from build123d import *

# Parameters (mm, degrees)
ESBO_O1_R                = 2.75
ESBO_O1_R_2              = 1.75
RESSALTO_EXTRUS_O1_DEPTH = 1
ESBO_O1_3_R              = 2.75
ESBO_O1_3_R_2            = 1.75
RESSALTO_EXTRUS_O2_DEPTH = 5
ESBO_O2_W                = 7
ESBO_O2_H                = 25
CORTE_EXTRUS_O1_DEPTH    = 6
CORTE_EXTRUS_O2_DEPTH    = 6
ESBO_O4_W                = 4
ESBO_O4_H                = 4
RESSALTO_EXTRUS_O3_DEPTH = 2


with BuildPart() as part:
    # Esboço1 → Ressalto-extrusão1 (new body)
    with BuildSketch(Plane.XY):
        with BuildLine():
            Line((23.75, 18.5), (-23.75, 18.5))
            ThreePointArc((-23.75, 18.5), (-21.805456352, 17.694543648), (-21, 15.75))
            ThreePointArc((-21, 15.75), (-23.75, 13), (-26.5, 15.75))
            Line((-26.5, 15.75), (-26.5, -15.75))
            ThreePointArc((-26.5, -15.75), (-23.75, -13), (-21, -15.75))
            ThreePointArc((-21, -15.75), (-21.805456352, -17.694543648), (-23.75, -18.5))
            Line((-23.75, -18.5), (23.75, -18.5))
            ThreePointArc((23.75, -18.5), (21.805456352, -13.805456352), (26.5, -15.75))
            Line((26.5, -15.75), (26.5, 15.75))
            ThreePointArc((26.5, 15.75), (21.805456352, 13.805456352), (23.75, 18.5))
        make_face()
        with Locations((23.75, 15.75)):
            Circle(ESBO_O1_R)
        with Locations((23.75, 15.75)):
            Circle(ESBO_O1_R_2, mode=Mode.SUBTRACT)
        with Locations((23.75, -15.75)):
            Circle(ESBO_O1_R)
        with Locations((23.75, -15.75)):
            Circle(ESBO_O1_R_2, mode=Mode.SUBTRACT)
        with Locations((-23.75, -15.75)):
            Circle(ESBO_O1_R)
        with Locations((-23.75, -15.75)):
            Circle(ESBO_O1_R_2, mode=Mode.SUBTRACT)
        with Locations((-23.75, 15.75)):
            Circle(ESBO_O1_R)
        with Locations((-23.75, 15.75)):
            Circle(ESBO_O1_R_2, mode=Mode.SUBTRACT)
    extrude(amount=RESSALTO_EXTRUS_O1_DEPTH)

    # Esboço1<3> → Ressalto-extrusão2 (add)
    with BuildSketch(Plane.XY):
        with Locations((-23.75, 15.75)):
            Circle(ESBO_O1_3_R)
        with Locations((-23.75, 15.75)):
            Circle(ESBO_O1_3_R_2, mode=Mode.SUBTRACT)
        with Locations((23.75, 15.75)):
            Circle(ESBO_O1_3_R)
        with Locations((23.75, 15.75)):
            Circle(ESBO_O1_3_R_2, mode=Mode.SUBTRACT)
        with Locations((23.75, -15.75)):
            Circle(ESBO_O1_3_R)
        with Locations((23.75, -15.75)):
            Circle(ESBO_O1_3_R_2, mode=Mode.SUBTRACT)
        with Locations((-23.75, -15.75)):
            Circle(ESBO_O1_3_R)
        with Locations((-23.75, -15.75)):
            Circle(ESBO_O1_3_R_2, mode=Mode.SUBTRACT)
    extrude(amount=RESSALTO_EXTRUS_O2_DEPTH)

    # Esboço2 → Corte-extrusão1 (cut)
    with BuildSketch(Plane.XY.offset(1)):
        with Locations((23, 0)):
            Rectangle(ESBO_O2_W, ESBO_O2_H)
    extrude(amount=-CORTE_EXTRUS_O1_DEPTH, mode=Mode.SUBTRACT)

    # Esboço3 → Corte-extrusão2 (cut)
    with BuildSketch(Plane(origin=(0, 0, 0), x_dir=(-1, 0, 0), z_dir=(0, 0, -1))):
        with BuildLine():
            Line((7.25, 12.814331343), (18.75, 12.814331343))
            Line((18.75, 12.814331343), (18.75, 8.814331343))
            Line((18.75, 8.814331343), (7.25, 8.814331343))
            ThreePointArc((7.25, 8.814331343), (6.75, 8.314331343), (7.25, 7.814331343))
            Line((7.25, 7.814331343), (19.75, 7.814331343))
            Line((19.75, 7.814331343), (19.75, 13.814331343))
            Line((19.75, 13.814331343), (7.25, 13.814331343))
            ThreePointArc((7.25, 13.814331343), (6.75, 13.314331343), (7.25, 12.814331343))
        make_face()
    extrude(amount=-CORTE_EXTRUS_O2_DEPTH, mode=Mode.SUBTRACT)

    # Esboço4 → Ressalto-extrusão3 (add)
    with BuildSketch(Plane.XY.offset(1)):
        with Locations((-16.75, 10.814331343)):
            Rectangle(ESBO_O4_W, ESBO_O4_H)
    extrude(amount=RESSALTO_EXTRUS_O3_DEPTH)


solid = part.part
Read the model definition and answer for the solid it produces. Units are mm, in the model's axes. A direction names the side the tool comes from. Coordinates: 2 decimals unless noted, no trailing zeros. Order: outer loops, then holes, each group sorted by start corner. A loop starts at its lowest first (then second) coordinate and runs counter-clockwise, first axis right, second up. Notation, with made-up numbers: (17.5, 29.5) -> (75.5, 29.5) arc R19 ccw to (75.5, 55.5) -> close; hole circle Ø10 at (-5, -26). An arc over 180 degrees is marked (long way). Answer as a JSON object with one key per item and string values.
1) A tool of negligible diameter and unlimited length cuts with its end or side. For faces 1 (the face through (23, -12.5, 0.5)), 2 (the face through (26.5, 14.1, 0.5)), 3 (the face through (-18.75, 11, 1)), 4 (the face through (-22, 15, 5)), 5 (the face through (-14.75, 11, 2)), from which of +Z, -Z, +X, -X, +Y, -Y can it reach the whole face along a straight path? Write none if from no direction.
Model answer:
{"face 1": "+Z, -Z, +X", "face 2": "+Z, -Z, +X, +Y, -Y", "face 3": "+Z, -Z", "face 4": "+Z, +X, -X, +Y, -Y", "face 5": "+Z, +X, +Y, -Y"}
2) Each of these flat-tipped pins is pushed along its axis until it touches: pin 1 (3 mm diameter, centred on x = -17.5, y = 11.5, fed in from +Z); pin 2 (1.1 mm diameter, centred on y = 10.5, z = 0.5, fed in from +X); pin 3 (1.5 mm diameter, centred on x = -10.5, z = 2, fed in from -Y); pin 4 (3 mm diameter, centred on x = 12, y = 7.5, fed in from +Z). Where does it stop, or does it pass through?
Model answer:
{"pin 1": "stops at z = 3", "pin 2": "stops at x = 19.5", "pin 3": "passes through", "pin 4": "stops at z = 1"}
3) A cutting plane is placed at A-A, the plane z = 2. State how many separate pieces and enclosed holes the cut face has, plus the area to 3 significant figures.
Model answer:
{"separate pieces": "5", "enclosed holes": "4", "area": "72.5 mm²"}
4) Consider line 1 along Y through (x, z) = (-23.75, 1.1); line 2 along Y through (x, z) = (-19.5, 0.7); line 3 along Z through (x, y) = (-2, 5). Determine where each line is inside the solid, lowest interval first. Write a range as from..to.
Model answer:
{"line 1": "y = -18.5..-17.5, -14..-13, 13..14, 17.5..18.5", "line 2": "y = -18.5..7.81, 13.81..18.5", "line 3": "z = 0..1"}
5) A cutting plane is placed at B-B, the plane y = 9.5. Determine the outline of the cut face in (x, z), plus the area to 3 significant figures.
Model answer:
{"outline": "(-26.5, 0) -> (-19.75, 0) -> (-19.75, 1) -> (-26.5, 1) -> close; (-18.75, 0) -> (19.5, 0) -> (19.5, 1) -> (-14.75, 1) -> (-14.75, 3) -> (-18.75, 3) -> close", "area": "53.0 mm²"}
6) The mould has two halves that part along Y. Classify faces 6 (the face through (-0.3, -18.5, 0.5)), 7 (the face through (-6.75, 13.33, 0.49)), 8 (the face through (-17, 11, 3)): released by +Y, released by -Y, zero draft, split by the parting line, or undercut.
Model answer:
{"face 6": "released by -Y", "face 7": "undercut", "face 8": "zero draft"}
